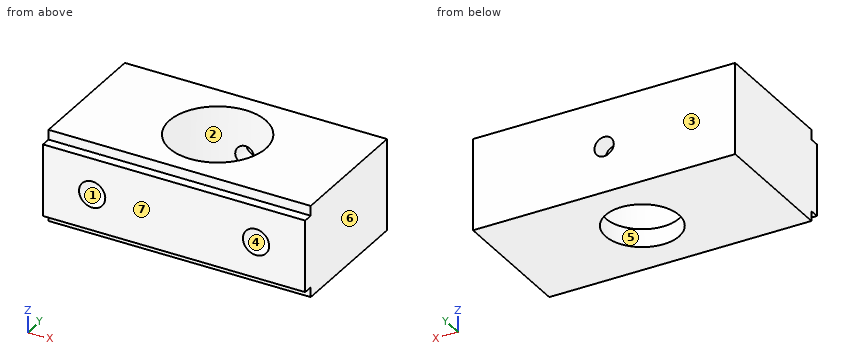
from build123d import *

# Parameters (mm, degrees)
SKETCH1_W                    = 69.088
SKETCH1_H                    = 37.45
EXTRUDE1_DEPTH               = 24.13
CUT_EXTRUDE1_DEPTH           = 8.128
CUT_EXTRUDE1_DEPTH_BACK      = 83.312
CUT_EXTRUDE4_DEPTH           = 25.4
CUT_EXTRUDE4_DEPTH_BACK      = 89.662
SKETCH11_W                   = 7.556551936
SKETCH11_H                   = 2.543
F_5_16_24_TAPPED_HOLE1_D     = 6.9088
F_5_16_24_TAPPED_HOLE1_DEPTH = 19.05254
F_5_16_24_TAPPED_HOLE1_TIP   = 2.075612922
CUT_EXTRUDE5_DEPTH           = 38.608
CUT_EXTRUDE5_DEPTH_BACK      = 11.938
SKETCH15_R                   = 12.72999994
SKETCH16_R                   = 14.7
SKETCH16_R_2                 = 9.7
BOSS_EXTRUDE1_DEPTH          = 4.73
F_1_4_20_TAPPED_HOLE2_D      = 5.1054
F_1_4_20_TAPPED_HOLE2_DEPTH  = 16.51
F_1_4_20_TAPPED_HOLE2_TIP    = 1.533816902


with BuildPart() as part:
    # Sketch1 → Extrude1 (new body)
    with BuildSketch(Plane.XY):
        with Locations((18.406260253, 9.092395655)):
            Rectangle(SKETCH1_W, SKETCH1_H)
    extrude(amount=EXTRUDE1_DEPTH)

    # Sketch2 → Cut-Extrude1 (cut, two sides: drawn at the far end of the back side and taken through both)
    with BuildSketch(Plane.ZY.offset(16.137739747).offset(-CUT_EXTRUDE1_DEPTH_BACK)):
        with BuildLine():
            Line((-1.394410139, -7.219604345), (2.59715, -7.219604345))
            Line((2.59715, -7.219604345), (2.59715, -10.370080057))
            Line((2.59715, -10.370080057), (21.53285, -10.370080057))
            Line((21.53285, -10.370080057), (21.53285, -7.219604345))
            Line((21.53285, -7.219604345), (26.024229083, -7.219604345))
            ThreePointArc((26.024229083, -7.219604345), (12.314909472, -19.255117467), (-1.394410139, -7.219604345))
        make_face()
    extrude(amount=CUT_EXTRUDE1_DEPTH + CUT_EXTRUDE1_DEPTH_BACK, mode=Mode.SUBTRACT)

    # Sketch11 → Cut-Extrude4 (cut, two sides: drawn at the far end of the back side and taken through both)
    with BuildSketch(Plane.ZY.offset(16.137739747).offset(-CUT_EXTRUDE4_DEPTH_BACK)):
        with Locations((-1.181125968, -8.361104345)):
            Rectangle(SKETCH11_W, SKETCH11_H)
        Polygon((21.534784946, -7.096819318), (21.532847251, -9.63981858), (29.089396994, -9.645576459), (29.091334688, -7.102577197), align=None)
    extrude(amount=CUT_EXTRUDE4_DEPTH + CUT_EXTRUDE4_DEPTH_BACK, mode=Mode.SUBTRACT)

    # 5/16-24 Tapped Hole1
    with Locations(Plane(origin=(-3.183739747, -9.632604345, 12.065), x_dir=(0, 0, -1), z_dir=(0, -1, 0))):
        with Locations((0, 0), (0, 43.18)):
            Hole(F_5_16_24_TAPPED_HOLE1_D / 2, depth=F_5_16_24_TAPPED_HOLE1_DEPTH)
            with Locations((0, 0, -(F_5_16_24_TAPPED_HOLE1_DEPTH + F_5_16_24_TAPPED_HOLE1_TIP / 2))):  # 118° drill point
                Cone(0, F_5_16_24_TAPPED_HOLE1_D / 2, F_5_16_24_TAPPED_HOLE1_TIP, mode=Mode.SUBTRACT)

    # Sketch15 → Cut-Extrude5 (cut, two sides: drawn at the far end of the back side and taken through both)
    with BuildSketch(Plane.XY.offset(-CUT_EXTRUDE5_DEPTH_BACK)):
        with Locations(Location((18.406260253, 10.317395655, 0), (0, 0, 180))):
            Circle(SKETCH15_R)
    extrude(amount=CUT_EXTRUDE5_DEPTH + CUT_EXTRUDE5_DEPTH_BACK, mode=Mode.SUBTRACT)

    # Sketch16 → Boss-Extrude1 (add)
    with BuildSketch(Plane.XY.offset(4.73)):
        with Locations((18.406260253, 10.317395655)):
            Circle(SKETCH16_R)
        with Locations((18.406260253, 10.317395655)):
            Circle(SKETCH16_R_2, mode=Mode.SUBTRACT)
    extrude(amount=-BOSS_EXTRUDE1_DEPTH)

    # 1/4-20 Tapped Hole2
    with Locations(Plane(origin=(18.406260253, 27.817395655, 12.065), x_dir=(0, 0, 1), z_dir=(0, 1, 0))):
        with Locations((0, 0)):
            Hole(F_1_4_20_TAPPED_HOLE2_D / 2, depth=F_1_4_20_TAPPED_HOLE2_DEPTH)
            with Locations((0, 0, -(F_1_4_20_TAPPED_HOLE2_DEPTH + F_1_4_20_TAPPED_HOLE2_TIP / 2))):  # 118° drill point
                Cone(0, F_1_4_20_TAPPED_HOLE2_D / 2, F_1_4_20_TAPPED_HOLE2_TIP, mode=Mode.SUBTRACT)


solid = part.part
For this review, take the finished solid that the model builds, in its own axes (mm). Face numbers are marked on the shaded views. A direction names the side the tool comes from. Coordinates: 2 decimals unless noted, no trailing zeros. Order: outer loops, then holes, each group sorted by start corner. A loop starts at its lowest first (then second) coordinate and runs counter-clockwise, first axis right, second up. Notation, with made-up numbers: (50, 4.25) - (71, 4.25) arc R27 ccw to (71, 43.25) - close; hole circle Ø2 at (-1.75, -17.5). An arc over 180 degrees is marked (long way). Answer as CSV lines item,"result". Start each with the question number.
1) Add section D-D (y = -3.5). State the section outline as (x, z) points (3 decimals), then the cut area to 3 significant figures.
2) Add section C-C (z = 7.75). State the section outline as (x, y) points.
3) Add section A-A (y = 16). State the section outline as (x, z) points (3 decimals).
4) Machinability: for the marked faces 1, 2 and 3, which of the approach directions +Z, -Z, +X, -X, +Y, -Y give a long, thin tool a straight path to every point of the face, cutting with its end or side? Answer none if there is none.
5) To check wall thickness, follow line 1 along X through (y, z) = (-0.5, 10.75); line 2 along X through (y, z) = (6, 12.75); line 3 along Z through (x, y) = (-3, 7). State the ranges of each line that lie inside material, in increasing order. Write a range as [from, to].
6) Insertion check: P1, Ø5.5, axis at x = -3.18, z = 12.06, coming from the -Y side; P2, Ø2.5, axis at x = 27.5, y = -9, coming from the +Z side; P3, Ø1.3, axis at x = 23, y = -8.5, coming from the -Z side. Each pin has a flat end and moves straight along its axis. Give the tip position at first contact, or say it passes through.
7) Draft analysis for pull direction X (two halves, no side actions). For the marked faces 4, 5, 6 and 7, state which applies: +X half, -X half, draft (parallel to the pull), parting line (faces both ways), or undercut.
Result:
1,outline,"(-16.138, 0) - (52.95, 0) - (52.95, 24.13) - (-16.138, 24.13) - close; hole circle Ø6.909 at (-3.184, 12.065); hole circle Ø6.909 at (39.996, 12.065)"
1,area,"1,590 mm^2"
2,outline,"(-16.14, -9.63) - (52.95, -9.63) - (52.95, 27.82) - (-16.14, 27.82) - close; hole circle Ø25.46 at (18.41, 10.32)"
3,outline,"(-16.138, 0) - (10.545, 0) - (10.545, 4.73) - (7.015, 4.73) - (7.015, 24.13) - (-16.138, 24.13) - close; (26.267, 0) - (52.95, 0) - (52.95, 24.13) - (29.798, 24.13) - (29.798, 4.73) - (26.267, 4.73) - close"
4,face 1,"-Y"
4,face 2,"+Z"
4,face 3,"+Z, -Z, +X, -X, +Y"
5,line 1,"[-16.14, -6.38], [0.01, 11.7], [25.12, 36.8], [43.19, 52.95]"
5,line 2,"[-16.14, -6.57], [0.2, 6.43], [30.38, 36.61], [43.38, 52.95]"
5,line 3,"[0, 8.62], [15.51, 24.13]"
6,P1,"y = 9.84"
6,P2,"z = 21.53"
6,P3,"z = 2.6"
7,face 4,"undercut"
7,face 5,"undercut"
7,face 6,"+X half"
7,face 7,"draft"
